Read the model definition and answer for the solid it produces. Units are mm, in the model's axes. Face numbers are marked on the shaded views. A direction names the side the tool comes from. Give positions to 0.01 mm unless a question says otherwise; leave off trailing zeros. Order: outer loops, then holes, each group sorted by start corner. A loop starts at its lowest first (then second) coordinate and runs counter-clockwise, first axis right, second up. Notation, with made-up numbers: (13, 56) - (71, 56) arc R22 ccw to (71, 71) - close; hole circle Ø5 at (-9.5, 56.5). An arc over 180 degrees is marked (long way). Use a Markdown table: item, result. Add a question column.
1. A cutting plane is placed at B-B on z = -20. Determine the outline of the cut face in (x, y).
2. Which of the six approach directions +Z, -Z, +X, -X, +Y, -Y give full straight-line access (tool end or side, diameter ignored) to the marked faces 4, 5, 6, 7 and 8?
3. For a pull along Y with two mould halves and no side action, classify the marked faces 1, 2 and 3 as released by +Y, released by -Y, zero draft, split by the parting line, or undercut.
4. A cutting plane is placed at C-C on y = -4. Determine the outline of the cut face in (x, z), and give its area (3 significant figures).
5. Flat-ended cylindrical pins translate along their axes: P1, Ø11, axis at x = 4, z = -26, coming from the +Y side; P2, Ø8, axis at x = 17.5, z = 4, coming from the -Y side; P3, Ø3, axis at x = -12.5, y = -3.5, coming from the -Z side; P4, Ø24, axis at x = 0, y = 0, coming from the +Z side. Find the tip coordinate at first contact, or state that the pin passes through.
6. A cutting plane is placed at A-A on x = 0. Determine the outline of the cut face in (y, z), and give its area (3 significant figures).
7. Consider L1, parallel to X at y = -0.85, z = -20; L2, parallel to Y at x = 0, z = 7.9; L3, parallel to Z at x = -24.5, y = 6.5. Determine where each line is inside the solid, lowest interval first.
8. A cutting plane is placed at D-D on x = -14. Determine the outline of the cut face in (y, z), and give its area (3 significant figures).
```python
from build123d import *

# Parameters (mm, degrees)
CROQUIS1_R              = 30
SALIENTE_EXTRUIR1_DEPTH = 10
CROQUIS2_W              = 60
CROQUIS2_H              = 40
SALIENTE_EXTRUIR2_DEPTH = 5
REDONDEO1_R             = 10
REDONDEO2_R             = 3
CROQUIS3_R              = 15
CORTAR_EXTRUIR1_DEPTH   = 5
CROQUIS4_R              = 10
CORTAR_EXTRUIR2_DEPTH   = 62.032778128
REDONDEO3_R             = 3


with BuildPart() as part:
    # Croquis1 → Saliente-Extruir1 (new body)
    with BuildSketch(Plane.XY):
        Circle(CROQUIS1_R)
    extrude(amount=SALIENTE_EXTRUIR1_DEPTH)

    # Croquis2 → Saliente-Extruir2 (add, symmetric)
    with BuildSketch(Plane(origin=(0, 0, 0), x_dir=(1, 0, 0), z_dir=(0, 1, 0))):
        with Locations((0, 20)):
            Rectangle(CROQUIS2_W, CROQUIS2_H)
    extrude(amount=SALIENTE_EXTRUIR2_DEPTH, both=True)

    # Redondeo1
    redondeo1_edges = [part.edges().sort_by_distance(p)[0] for p in [
        (-30, 0, -40),
        (30, 0, -40),
    ]]
    fillet(redondeo1_edges, radius=REDONDEO1_R)

    # Redondeo2
    # the kernel refuses this fillet: 3 mm, written as the material it takes off along each edge
    with BuildSketch(Plane(origin=(30, -5, 0), x_dir=(0, 1, 0), z_dir=(0, 0, -1)), Plane(origin=(30, 5, 0), x_dir=(-1, 0, 0), z_dir=(0, 0, -1)), Plane(origin=(-30, -5, -30), x_dir=(0, 1, 0), z_dir=(0, 0, 1)), Plane(origin=(-30, 5, -30), x_dir=(1, 0, 0), z_dir=(0, 0, 1))) as redondeo2_piece_1:
        with BuildLine():
            CenterArc((REDONDEO2_R, -REDONDEO2_R), REDONDEO2_R, 90, 90)
            Line((0, -REDONDEO2_R), (0, 0))
            Line((0, 0), (REDONDEO2_R, 0))
        make_face()
    extrude(amount=30, mode=Mode.SUBTRACT)
    with BuildSketch(Plane(origin=(20, -5, -40), x_dir=(0, 1, 0), z_dir=(-1, 0, 0)), Plane(origin=(20, 5, -40), x_dir=(0, 0, 1), z_dir=(-1, 0, 0))) as redondeo2_piece_2:
        with BuildLine():
            CenterArc((REDONDEO2_R, -REDONDEO2_R), REDONDEO2_R, 90, 90)
            Line((0, -REDONDEO2_R), (0, 0))
            Line((0, 0), (REDONDEO2_R, 0))
        make_face()
    extrude(amount=40, mode=Mode.SUBTRACT)
    with BuildSketch(Plane(origin=(-20, -5, -30), x_dir=(-1, 0, 0), z_dir=(0, 0, 1))) as redondeo2_piece_3:
        with BuildLine():
            CenterArc((10 - REDONDEO2_R, -REDONDEO2_R), REDONDEO2_R, 0, 90)
            Line((10 - REDONDEO2_R, 0), (10, 0))
            Line((10, 0), (10, -REDONDEO2_R))
        make_face()
    revolve(axis=Axis((-20, -5, -30), (0, -1, 0)), revolution_arc=90, mode=Mode.SUBTRACT)
    with BuildSketch(Plane(origin=(20, -5, -30), x_dir=(1, 0, 0), z_dir=(0, 0, 1))) as redondeo2_piece_4:
        with BuildLine():
            CenterArc((10 - REDONDEO2_R, REDONDEO2_R), REDONDEO2_R, 270, 90)
            Line((10 - REDONDEO2_R, 0), (10, 0))
            Line((10, 0), (10, REDONDEO2_R))
        make_face()
    revolve(axis=Axis((20, -5, -30), (0, 1, 0)), revolution_arc=90, mode=Mode.SUBTRACT)
    with BuildSketch(Plane(origin=(-20, 5, -30), x_dir=(-1, 0, 0), z_dir=(0, 0, 1))) as redondeo2_piece_5:
        with BuildLine():
            CenterArc((10 - REDONDEO2_R, REDONDEO2_R), REDONDEO2_R, 270, 90)
            Line((10, REDONDEO2_R), (10, 0))
            Line((10, 0), (10 - REDONDEO2_R, 0))
        make_face()
    revolve(axis=Axis((-20, 5, -30), (0, -1, 0)), revolution_arc=90, mode=Mode.SUBTRACT)
    with BuildSketch(Plane(origin=(20, 5, -30), x_dir=(1, 0, 0), z_dir=(0, 0, 1))) as redondeo2_piece_6:
        with BuildLine():
            CenterArc((10 - REDONDEO2_R, -REDONDEO2_R), REDONDEO2_R, 0, 90)
            Line((10, -REDONDEO2_R), (10, 0))
            Line((10, 0), (10 - REDONDEO2_R, 0))
        make_face()
    revolve(axis=Axis((20, 5, -30), (0, 1, 0)), revolution_arc=90, mode=Mode.SUBTRACT)

    # Croquis3 → Cortar-Extruir1 (cut)
    with BuildSketch(Plane.XY.offset(10)):
        Circle(CROQUIS3_R)
    extrude(amount=-CORTAR_EXTRUIR1_DEPTH, mode=Mode.SUBTRACT)

    # Croquis4 → Cortar-Extruir2 (cut, through all)
    with BuildSketch(Plane.XZ.offset(5)):
        with Locations(Location((0, -20, 0), (0, 0, 270))):
            Circle(CROQUIS4_R)
    extrude(amount=-CORTAR_EXTRUIR2_DEPTH, mode=Mode.SUBTRACT)

    # Redondeo3
    redondeo3_edges = [part.edges().sort_by_distance(p)[0] for p in [
        (0, 5, -10),
        (0, -5, -10),
    ]]
    fillet(redondeo3_edges, radius=REDONDEO3_R)


solid = part.part
```
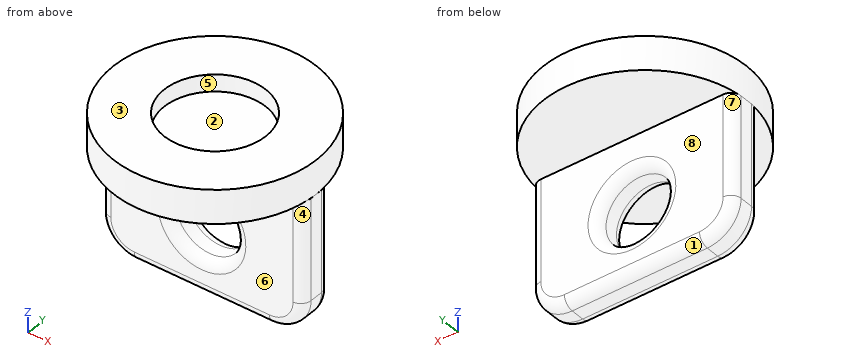
Output values:
| question | item | result |
|---|---|---|
| 1 | outline | (-30, -2) arc R3 ccw to (-27, -5) - (-13, -5) arc R3 ccw to (-10, -2) - (-10, 2) arc R3 ccw to (-13, 5) - (-27, 5) arc R3 ccw to (-30, 2) - close; (10, -2) arc R3 ccw to (13, -5) - (27, -5) arc R3 ccw to (30, -2) - (30, 2) arc R3 ccw to (27, 5) - (13, 5) arc R3 ccw to (10, 2) - close |
| 2 | face 4 | -Z, +X, -Y |
| 2 | face 5 | +Z |
| 2 | face 6 | -Z, +X, -X, -Y |
| 2 | face 7 | -Z, -X, +Y |
| 2 | face 8 | -Z, +X, -X, +Y |
| 3 | face 1 | released by +Y |
| 3 | face 2 | undercut |
| 3 | face 3 | zero draft |
| 4 | outline | (-29.73, 0) - (-29.24, 0) - (-29.24, -30) arc R9.24 ccw to (-20, -39.24) - (20, -39.24) arc R9.24 ccw to (29.24, -30) - (29.24, 0) - (29.73, 0) - (29.73, 10) - (14.46, 10) - (14.46, 5) - (-14.46, 5) - (-14.46, 10) - (-29.73, 10) - close; hole circle Ø21.53 at (0, -20) |
| 4 | area | 2,340 mm² |
| 5 | P1 | y = 4.99 |
| 5 | P2 | y = -26.79 |
| 5 | P3 | z = -40 |
| 5 | P4 | z = 5 |
| 6 | outline | (-30, 0) - (-5, 0) - (-5, -7) arc R3 ccw to (-2, -10) - (2, -10) arc R3 ccw to (5, -7) - (5, 0) - (30, 0) - (30, 10) - (15, 10) - (15, 5) - (-15, 5) - (-15, 10) - (-30, 10) - close; (-5, -37) arc R3 ccw to (-2, -40) - (2, -40) arc R3 ccw to (5, -37) - (5, -33) arc R3 ccw to (2, -30) - (-2, -30) arc R3 ccw to (-5, -33) - close |
| 6 | area | 638 mm² |
| 7 | L1 | -30 to -10, 10 to 30 |
| 7 | L2 | -30 to -15, 15 to 30 |
| 7 | L3 | 0 to 10 |
| 8 | outline | (-26.53, 0) - (-5, 0) - (-5, -37) arc R3 ccw to (-2, -40) - (2, -40) arc R3 ccw to (5, -37) - (5, 0) - (26.53, 0) - (26.53, 10) - (5.39, 10) - (5.39, 5) - (-5.39, 5) - (-5.39, 10) - (-26.53, 10) - close |
| 8 | area | 873 mm² |
